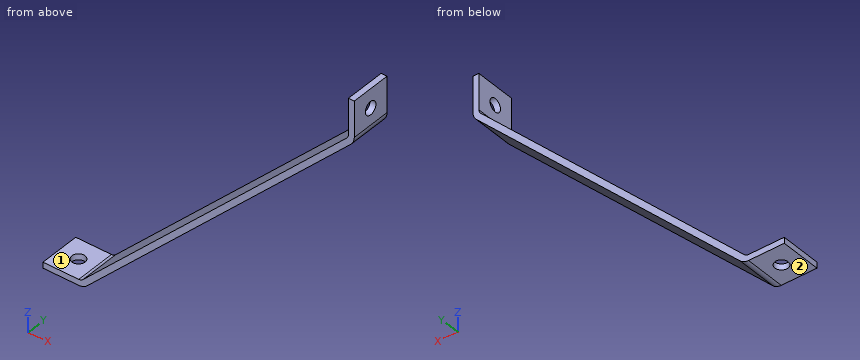
```python
from build123d import *

# Parameters (mm, degrees)
F1_DEPTH = 22.225
F2_R     = 6.35
F3_R     = 12.7
F4_R     = 7.14375
F5_DEPTH = 25.4
F6_R     = 7.14375
F7_DEPTH = 206.502


with BuildPart() as f1:
    # F0 (on Front) → F1 (new body, symmetric)
    with BuildSketch(Plane.XZ):
        Polygon((-168.275, -168.275), (-124.369744, -168.275), (-124.097372, -168.002628), (168.002628, 124.097372), (168.275, 124.369744), (168.275, 168.275), (161.925, 168.275), (161.925, 127), (-127, -161.925), (-168.275, -161.925), align=None)
    extrude(amount=F1_DEPTH, both=True)

    # F2
    f2_edges = [f1.edges().sort_by_distance(p)[0] for p in [
        (-127, 0, -161.925),
        (161.925, 0, 127),
    ]]
    fillet(f2_edges, radius=F2_R)

    # F3
    f3_edges = [f1.edges().sort_by_distance(p)[0] for p in [
        (-124.369744, 0, -168.275),
        (168.275, 0, 124.369744),
    ]]
    fillet(f3_edges, radius=F3_R)

    # F4 (on face) → F5 (cut)
    with BuildSketch(Plane(origin=(161.925, 0, 0), x_dir=(0, -1, 0), z_dir=(-1, 0, 0))):
        with Locations((0, 147.6248)):
            Circle(F4_R)
    extrude(amount=-F5_DEPTH, mode=Mode.SUBTRACT)

    # F6 (on Top) → F7 (cut)
    with BuildSketch(Plane.XY):
        with Locations((-147.6248, 0)):
            Circle(F6_R)
    extrude(amount=-F7_DEPTH, mode=Mode.SUBTRACT)


solid = f1.part
```
Here's how the part is built. I have some questions about the finished solid (model axes, mm). Face numbers are marked on the shaded views. A direction names the side the tool comes from. Round coordinates to 2 decimals unless told otherwise and drop trailing zeros. Write each loop counter-clockwise with the first axis right and the second up, starting at its lowest first coordinate (ties: lowest second). Pieces come first, ordered by that corner, then holes.
Q1. Please list where these lines run through material, in increasing order: probe 1 along Z at (x, y) = (166.5, 0) (3 decimals); probe 2 along Z at (x, y) = (164, 0) (3 decimals); probe 3 along X at (y, z) = (-15, -37) (3 decimals).
Q2. Which directions (+Z, -Z, +X, -X, +Y, -Y) give clear straight access to the entire face, cutting with the end or side of a thin tool? Please do the marked faces 1 and 2.
Q3. If we section it at A-A on y = 0: Write out the boundary of the cut face in (x, z) (3 decimals), plus the area to 3 significant figures.
Q4. If we section it at C-C on z = -30: Write out the boundary of the cut face in (x, y) (3 decimals).
Q5. Will these pins go through, and if not, where does the flat tip stop? P1, Ø8, axis at x = -57.5, y = -17.5, coming from the -Z side; P2, Ø12, axis at x = -4, y = 8.5, coming from the -Z side; P3, Ø6, axis at x = -24.5, y = 15, coming from the +Z side (3 decimals); P4, Ø11.5, axis at y = 0, z = 147.62, coming from the +X side.
Q6. If we section it at B-B on x = 28.5: Write out the boundary of the cut face in (y, z) (3 decimals).
Answer below:
1. probe 1: z = 123.155 to 140.481, 154.769 to 168.275
1. probe 2: z = 120.095 to 140.481, 154.769 to 168.275
1. probe 3: x = -2.075 to 6.905
2. face 1: +Z, -X, +Y, -Y
2. face 2: -Z, +X, -X, +Y, -Y
3. outline: (-168.275, -168.275) - (-154.769, -168.275) - (-154.769, -161.925) - (-168.275, -161.925) - close; (-140.481, -168.275) - (-129.63, -168.275) arc R12.7 ccw to (-120.65, -164.555) - (164.555, 120.65) arc R12.7 ccw to (168.275, 129.63) - (168.275, 140.481) - (161.925, 140.481) - (161.925, 129.63) arc R6.35 cw to (160.065, 125.14) - (-125.14, -160.065) arc R6.35 cw to (-129.63, -161.925) - (-140.481, -161.925) - close; (161.925, 154.769) - (168.275, 154.769) - (168.275, 168.275) - (161.925, 168.275) - close
3. area: 2,970 mm2
4. outline: (4.925, -22.225) - (13.905, -22.225) - (13.905, 22.225) - (4.925, 22.225) - close
5. P1: stops at z = -105.41
5. P2: stops at z = -53.91
5. P3: stops at z = -56.425
5. P4: passes through
6. outline: (-22.225, -15.405) - (22.225, -15.405) - (22.225, -6.425) - (-22.225, -6.425) - close
